```python
from build123d import *

# Parameters (mm, degrees)
BOSS_EXTRUDE1_DEPTH      = 6.35
FILLET1_R                = 2.54
FILLET2_R                = 2.54
F_0_257_DIAMETER_HOLE1_D = 6.5278


with BuildPart() as part:
    # Sketch1 → Boss-Extrude1 (new body)
    with BuildSketch(Plane.XY):
        Polygon((-6.35, 0), (0, 0), (44.45, 0), (44.45, 32.01), (44.45, 44.19), (44.45, 50.8), (0, 50.8), (0, 76.2), (-50.8, 76.2), (-50.8, 50.8), align=None)
        Polygon((-12.7, 22.225), (-38.1, 50.8), (-12.7, 50.8), align=None, mode=Mode.SUBTRACT)
        with BuildLine():
            ThreePointArc((0.26, 6.35), (-0.183847763, 6.166152237), (0, 6.61))
            Line((0, 6.61), (0, 18.79))
            ThreePointArc((0, 18.79), (-0.183847763, 19.233847763), (0.26, 19.05))
            Line((0.26, 19.05), (6.09, 19.05))
            ThreePointArc((6.09, 19.05), (6.533847763, 19.233847763), (6.35, 18.79))
            Line((6.35, 18.79), (6.35, 6.61))
            ThreePointArc((6.35, 6.61), (6.533847763, 6.166152237), (6.09, 6.35))
            Line((6.09, 6.35), (0.26, 6.35))
        make_face(mode=Mode.SUBTRACT)
        with BuildLine():
            Line((31.75, 6.61), (31.75, 18.79))
            ThreePointArc((31.75, 18.79), (31.566152237, 19.233847763), (32.01, 19.05))
            Line((32.01, 19.05), (37.84, 19.05))
            ThreePointArc((37.84, 19.05), (38.283847763, 19.233847763), (38.1, 18.79))
            Line((38.1, 18.79), (38.1, 6.61))
            ThreePointArc((38.1, 6.61), (38.283847763, 6.166152237), (37.84, 6.35))
            Line((37.84, 6.35), (32.01, 6.35))
            ThreePointArc((32.01, 6.35), (31.566152237, 6.166152237), (31.75, 6.61))
        make_face(mode=Mode.SUBTRACT)
        with BuildLine():
            ThreePointArc((0, 44.19), (-0.183847763, 44.633847763), (0.26, 44.45))
            Line((0.26, 44.45), (6.09, 44.45))
            ThreePointArc((6.09, 44.45), (6.533847763, 44.633847763), (6.35, 44.19))
            Line((6.35, 44.19), (6.35, 32.01))
            ThreePointArc((6.35, 32.01), (6.533847763, 31.566152237), (6.09, 31.75))
            Line((6.09, 31.75), (0.26, 31.75))
            ThreePointArc((0.26, 31.75), (-0.183847763, 31.566152237), (0, 32.01))
            Line((0, 32.01), (0, 44.19))
        make_face(mode=Mode.SUBTRACT)
        with BuildLine():
            Line((38.1, 44.19), (38.1, 32.01))
            ThreePointArc((38.1, 32.01), (38.283847763, 31.566152237), (37.84, 31.75))
            Line((37.84, 31.75), (32.01, 31.75))
            ThreePointArc((32.01, 31.75), (31.566152237, 31.566152237), (31.75, 32.01))
            Line((31.75, 32.01), (31.75, 44.19))
            ThreePointArc((31.75, 44.19), (31.566152237, 44.633847763), (32.01, 44.45))
            Line((32.01, 44.45), (37.84, 44.45))
            ThreePointArc((37.84, 44.45), (38.283847763, 44.633847763), (38.1, 44.19))
        make_face(mode=Mode.SUBTRACT)
    extrude(amount=BOSS_EXTRUDE1_DEPTH)

    # Fillet1
    fillet1_edges = [part.edges().sort_by_distance(p)[0] for p in [
        (44.45, 0, 3.175),
        (-6.35, 0, 3.175),
        (-50.8, 50.8, 3.175),
        (-50.8, 76.2, 3.175),
        (0, 76.2, 3.175),
        (0, 50.8, 3.175),
        (44.45, 50.8, 3.175),
    ]]
    fillet(fillet1_edges, radius=FILLET1_R)

    # Fillet2
    fillet2_edges = [part.edges().sort_by_distance(p)[0] for p in [
        (-12.7, 22.225, 3.175),
        (-12.7, 50.8, 3.175),
        (-38.1, 50.8, 3.175),
    ]]
    fillet(fillet2_edges, radius=FILLET2_R)

    # F (0.257) Diameter Hole1 (through all)
    with Locations(Plane.XY.offset(6.35)):
        with Locations((-38.1, 63.44747919), (-12.7, 63.44747919)):
            Hole(F_0_257_DIAMETER_HOLE1_D / 2)


solid = part.part
```
The listing builds one solid part. Answer for the finished solid, in the listing's coordinates (mm). A direction names the side the tool comes from. Give positions to 0.01 mm unless a question says otherwise; leave off trailing zeros. Loops run counter-clockwise (first coordinate to the right, second up) from the corner with the lowest first, then second, coordinate; pieces in that order, holes last. Notation, with made-up numbers: (23.5, -33.5) - (61.5, -33.5) arc R37 ccw to (61.5, 3.5) - close; hole circle Ø10 at (76, 23.5). An arc over 180 degrees is marked (long way). Return JSON: item names as keys, results as strings. Group by question number.
1. Determine the mould class of faces 3 (the flat face through (-28.94, 25.82, 3.13)), 4 (the flat face through (35, 31.75, 3)), 5 (the cylindrical face through (43.686, 0.724, 3.219)), 6 (the flat face through (18, 0, 3)) for opening direction X: pulls with the +X half, pulls with the -X half, needs draft (parallel to the pull), parting line crosses it, or undercut.
2. Find section A-A (y = 39). Write down the section's boundary in (x, z) (3 decimals), then the cut area to 3 significant figures.
3. Which of the six approach directions +Z, -Z, +X, -X, +Y, -Y give full straight-line access (tool end or side, diameter ignored) to faces 1 (the cylindrical face through (43.726, 50.036, 3.219)), 2 (the flat face through (3, 19.05, 3))?
4. Find section B-B (y = 62). Write down the section's boundary in (x, z).
5. Find section C-C (x = 20). Write down the section's boundary in (y, z), then the cut area to 3 significant figures.
6. Straight lines are drawn through the part: line 1 (Y direction, x = 37, z = 4); line 2 (X direction, y = 33.5, z = 2.5); line 3 (Y direction, x = 32, z = 2.5). For each, find the intervals that lie inside material, in ascending order. Write a range as [from, to].
7. Given pin 1 Ø3 at (y, z) = (40, 4) entering from -X; pin 2 Ø3 at (x, z) = (-21, 3) entering from -Y; pin 3 Ø1.9 at (y, z) = (15, 5) entering from -X, each flat-ended and moving along its own axis, determine where each tip first touches the part or whether it passes through.
8. Find section D-D (z = 4). State how many separate pieces and enclosed holes the cut face has, then the cut area to 3 significant figures.
Verdict:
{
 "1": {"face 3": "pulls with the -X half", "face 4": "undercut", "face 5": "pulls with the +X half", "face 6": "needs draft"},
 "2": {"outline": "(-40.475, 0) - (-27.611, 0) - (-27.611, 6.35) - (-40.475, 6.35) - close; (-12.7, 0) - (0, 0) - (0, 6.35) - (-12.7, 6.35) - close; (6.35, 0) - (31.75, 0) - (31.75, 6.35) - (6.35, 6.35) - close; (38.1, 0) - (44.45, 0) - (44.45, 6.35) - (38.1, 6.35) - close", "area": "364 mm^2"},
 "3": {"face 1": "+Z, -Z, +X, +Y", "face 2": "+Z, -Z"},
 "4": {"outline": "(-50.8, 0) - (-41.03, 0) - (-41.03, 6.35) - (-50.8, 6.35) - close; (-35.17, 0) - (-15.63, 0) - (-15.63, 6.35) - (-35.17, 6.35) - close; (-9.77, 0) - (0, 0) - (0, 6.35) - (-9.77, 6.35) - close"},
 "5": {"outline": "(0, 0) - (50.8, 0) - (50.8, 6.35) - (0, 6.35) - close", "area": "323 mm^2"},
 "6": {"line 1": "y = [0, 6.35], [19.05, 31.75], [44.45, 50.8]", "line 2": "x = [-35.66, -22.72], [-12.7, 0], [6.35, 31.75], [38.1, 44.45]", "line 3": "y = [0, 6.28], [19.12, 31.68], [44.52, 50.8]"},
 "7": {"pin 1": "stops at x = -42.66", "pin 2": "stops at y = 15.03", "pin 3": "stops at x = -20.31"},
 "8": {"separate pieces": "1", "enclosed holes": "7", "area": "4,260 mm^2"}
}
